```python
from build123d import *

# Parameters (mm, degrees)
PAD011_DEPTH    = 6
SKETCH019_W     = 4
SKETCH019_H     = 4
POCKET002_DEPTH = 3.451
PAD012_DEPTH    = 2.5
FILLET004_R     = 0.3


with BuildPart() as part:
    # Sketch018 → Pad011 (new body, symmetric)
    with BuildSketch(Plane.YZ):
        with BuildLine():
            Line((13.1, -7.9), (13.1, -3.9))
            Line((13.1, -3.9), (16.95, -3.9))
            Line((16.95, -3.9), (16.95, -4.9))
            Line((16.95, -4.9), (16.75, -4.9))
            Line((16.75, -4.9), (16.75, -4.5))
            Line((16.75, -4.5), (16.55, -4.3))
            Line((16.55, -4.3), (13.8, -4.3))
            ThreePointArc((13.8, -4.3), (13.587868, -4.387868), (13.5, -4.6))
            Line((13.5, -4.6), (13.5, -7.2))
            ThreePointArc((13.5, -7.2), (13.587868, -7.412132), (13.8, -7.5))
            Line((13.8, -7.5), (16.5, -7.5))
            Line((16.5, -7.5), (16.7, -7.3))
            Line((16.7, -7.3), (16.7, -7.1))
            Line((16.7, -7.1), (16.9, -7.1))
            Line((16.9, -7.1), (16.9, -7.5))
            Line((16.5, -7.9), (16.9, -7.5))
            Line((16.5, -7.9), (13.1, -7.9))
        make_face()
    extrude(amount=PAD011_DEPTH, both=True)

    # Sketch019 (on Face10 of Pad011) → Pocket002 (cut, through all)
    with BuildSketch(Plane.ZX.offset(13.5)):
        with Locations((-7.9, 0)):
            Rectangle(SKETCH019_W, SKETCH019_H)
    extrude(amount=POCKET002_DEPTH, mode=Mode.SUBTRACT)

    # Sketch020 → Pad012 (join, symmetric)
    with BuildSketch(Plane.YZ):
        with BuildLine():
            Line((13.1, -3.9), (12, -3.9))
            ThreePointArc((12, -3.9), (11.717157, -4.017157), (11.6, -4.3))
            Line((11.6, -4.3), (11.6, -7.5))
            ThreePointArc((11.6, -7.5), (11.717157, -7.782843), (12, -7.9))
            Line((12, -7.9), (13.1, -7.9))
            Line((13.1, -7.9), (13.1, -7.5))
            Line((12, -7.5), (13.1, -7.5))
            Line((12, -4.3), (12, -7.5))
            Line((13.1, -4.3), (12, -4.3))
            Line((13.1, -4.3), (13.1, -3.9))
        make_face()
    extrude(amount=PAD012_DEPTH, both=True)

    # Fillet004
    fillet004_edges = [part.edges().sort_by_distance(p)[0] for p in [
        (0, 12, -4.3),
        (0, 12, -7.5),
        (0, 13.1, -7.5),
        (0, 13.1, -4.3),
    ]]
    fillet(fillet004_edges, radius=FILLET004_R)


solid = part.part
```
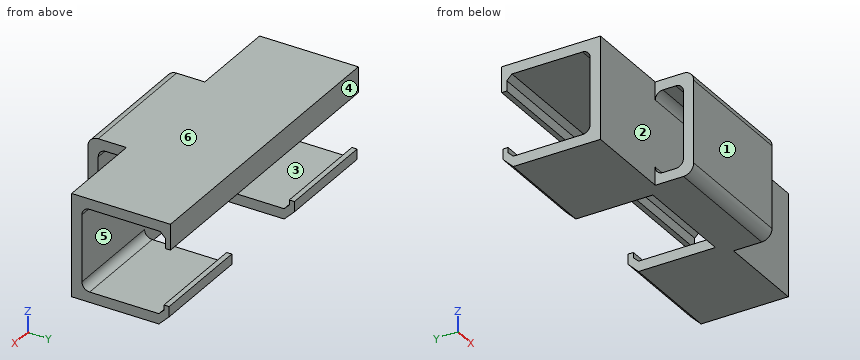
CAD build for the part. Positions are in the model's coordinates, mm. Face numbers are marked on the shaded views. A direction names the side the tool comes from. Coordinates: 2 decimals unless noted, no trailing zeros. Order: outer loops, then holes, each group sorted by start corner. A loop starts at its lowest first (then second) coordinate and runs counter-clockwise, first axis right, second up. Notation, with made-up numbers: (66, 30.5) -> (125, 30.5) arc R30 cw to (125, 58.5) -> close; hole circle Ø9 at (-10, 88.25). An arc over 180 degrees is marked (long way). Use one line per item in the form item = value. Start each with the question number.
1) Band-saw the part on D-D on z = -5.9. Give the cut face in (x, y), then the cut area to 3 significant figures.
2) Band-saw the part on B-B on y = 12.5. Give the cut face in (x, z).
3) Drill centre lines: L1, parallel to Z at x = -2.25, y = 12.6; L2, parallel to Y at x = -4.5, z = -4.65; L3, parallel to Y at x = -2, z = -4.75. Where is each one in solid material? Low to high. Write a range as [from, to].
4) Band-saw the part on A-A on y = 15.6. Give the cut face in (x, z).
5) Band-saw the part on C-C on x = 1.75. Give the cut face in (y, z).
6) Tool access for the marked faces 1, 2 and 3: list every direction of +Z, -Z, +X, -X, +Y, -Y with a clear straight run to the whole face (end or side of a thin tool).
7) Pull direction Z, two halves, no side cores. Call the marked faces 4, 5 and 6: +Z half, -Z half, draft (parallel to the pull), parting line (faces both ways), or undercut.
Entries:
q1.outline = (-6, 13.1) -> (6, 13.1) -> (6, 13.5) -> (-6, 13.5) -> close; (-2.5, 11.6) -> (2.5, 11.6) -> (2.5, 12) -> (-2.5, 12) -> close
q1.area = 6.80 mm2
q2.outline = (-2.5, -7.9) -> (2.5, -7.9) -> (2.5, -7.5) -> (-2.5, -7.5) -> close; (-2.5, -4.3) -> (2.5, -4.3) -> (2.5, -3.9) -> (-2.5, -3.9) -> close
q3.L1 = [-7.9, -7.5], [-4.3, -3.9]
q3.L2 = [13.1, 13.5], [16.75, 16.95]
q3.L3 = [11.6, 12], [13.1, 13.5], [16.75, 16.95]
q4.outline = (-6, -7.9) -> (-2, -7.9) -> (-2, -7.5) -> (-6, -7.5) -> close; (-6, -4.3) -> (6, -4.3) -> (6, -3.9) -> (-6, -3.9) -> close; (2, -7.9) -> (6, -7.9) -> (6, -7.5) -> (2, -7.5) -> close
q5.outline = (11.6, -7.5) arc R0.4 ccw to (12, -7.9) -> (13.5, -7.9) -> (13.5, -4.6) arc R0.3 cw to (13.8, -4.3) -> (16.55, -4.3) -> (16.75, -4.5) -> (16.75, -4.9) -> (16.95, -4.9) -> (16.95, -3.9) -> (12, -3.9) arc R0.4 ccw to (11.6, -4.3) -> close; hole (12, -7.2) arc R0.3 ccw to (12.3, -7.5) -> (12.8, -7.5) arc R0.3 ccw to (13.1, -7.2) -> (13.1, -4.6) arc R0.3 ccw to (12.8, -4.3) -> (12.3, -4.3) arc R0.3 ccw to (12, -4.6) -> close
q6.face_1 = +Z, -Z, +X, -X, -Y
q6.face_2 = none
q6.face_3 = +X, -X
q7.face_4 = draft
q7.face_5 = undercut
q7.face_6 = +Z half
